Autodesk Inventor part; units mm, degrees
ref_plane "YZ Plane" through (0, 0, 0) normal (1, 0, 0) x (0, 1, 0)
ref_plane "XZ Plane" through (0, 0, 0) normal (0, 1, 0) x (-1, 0, 0)
ref_plane "XY Plane" through (0, 0, 0) normal (0, 0, 1) x (1, 0, 0)
sketch "Sketch1" plane through (0, 0, 0) normal (1, 0, 0) x (0, 1, 0)
  circle A0 centre (0, 0) radius 6
  line L0 (36, -46) -> (36, 34)
  line L1 (36, 34) -> (-29, 34)
  line L2 (-29, 34) -> (-29, -46)
  line L3 (-29, -46) -> (36, -46)
  point P0 (0, -17.5)
  point P1 (17.5, 0)
  point P2 (0, 17.5)
  point P3 (-17.5, 0)
  point P4 (0, -30)
  point P5 (0, 30)
  point P6 (31, -41)
  point P7 (31, 29)
  point P8 (-24, 29)
  point P9 (-24, -41)
  dimension "d6" = 30
  dimension "d9" = 360
  dimension "d15" = 5
  dimension "d16" = 5
  dimension "d17" = 80
  dimension "d18" = 65
  dimension "d28" = 5
  dimension "d29" = 55
  dimension "d30" = 55
  dimension "d38" = 12
extrude "Extrusion1" add sketch "Sketch1" along normal blind 2
hole "Hole1" at (0, 31, -41) at (0, 31, 29) at (0, -24, 29) at (0, -24, -41) direction (1, 0, 0) diameter 3.2 depth 43.75 tip angle 118
sketch "Sketch2" plane through (0, 0, 0) normal (-1, 0, 0) x (0, 0, 1)
  circle A0 centre (-40, 0) radius 6
  line L0 (-46, 36) -> (34, 36)
  line L1 (-46, 36) -> (-52, 36)
  line L2 (-52, 36) -> (-52, -29)
  line L3 (-52, -29) -> (-46, -29)
  line L4 (-46, -29) -> (-46, 36)
  point P0 (0, 0)
  point P1 (0, 25.1294)
  point P2 (0, -32.6005)
  dimension "d31" = 40
  dimension "d32" = 12
  dimension "d33" = 6
extrude "Extrusion2" add sketch "Sketch2" against normal blind 2 contours L4 L3 L2 L1
extrude "Extrusion3" cut sketch "Sketch2" against normal blind 2 contours A0
sketch "Sketch3" plane through (0, 0, 0) normal (-1, 0, 0) x (0, 0, 1)
  line L0 (34, 36) -> (34, -29)
  line L1 (34, 36) -> (46, 36)
  line L2 (46, 36) -> (46, -29)
  line L3 (46, -29) -> (34, -29)
  line L4 (34, -29) -> (34, 36)
  line L5 (-52, 36) -> (-52, -29)
  line L6 (-52, 36) -> (-82, 36)
  line L7 (-82, 36) -> (-82, -29)
  line L8 (-82, -29) -> (-52, -29)
  line L9 (-52, -29) -> (-52, 36)
  circle A0 centre (0, 0) radius 6
  circle A1 centre (0, 0) radius 15.315
  circle A2 centre (-40, 0) radius 6
  circle A3 centre (-40, 0) radius 15.315
  line L10 (-40, 15.315) -> (-90.0791, 8.5618)
  line L11 (-35.9433, -14.768) -> (-79.6302, -20.6591)
  line L12 (0, 15.315) -> (59.9492, 7.4438)
  line L13 (-3.9709, -14.9288) -> (55.9782, -22.7999)
  circle A4 centre (29, 15.315) radius 1.6
  point P0 (-71.9486, -24)
  point P1 (-71.9486, 13.715)
  point P2 (-52, -29)
  dimension "d41" = 30.63
  dimension "d39" = 12
  dimension "d40" = 30
  dimension "d42" = 30.63
  dimension "d43" = 7.68
  dimension "d44" = 0
  dimension "d45" = 7.48
extrude "Extrusion4" add sketch "Sketch3" against normal blind 2 contours L1 L2 L12 L0 | L12 L2 L13 L0 | L13 L2 L3 L0 | L5 L10 L7 L6 | L5 A3 L8 L7 L10 | L5 A3
hole "Hole2" at (0, -24, -71.9486) at (0, 13.715, -71.9486) at (0, 15.315, 29) direction (1, 0, 0) diameter 3.2 depth 43.75 tip angle 118
fillet "Fillet1" radius 8.25 4 edges at (1, 36, -82) (1, -29, -82) (1, -29, 46) (1, 36, 46)
sketch "Sketch4" plane through (0, 0, 0) normal (-1, 0, 0) x (0, 0, 1)
  line L0 (46, -20.75) -> (46, 27.75)
  point P0 (0, 0)
  point P1 (46, 0)
hole "Hole3" at (0, 0, 46) direction (1, 0, 0) diameter 3.2 depth 43.75 tip angle 118
fillet "Fillet2" radius 2 2 edges at (1, 1.6, 46) (1, -1.6, 46)
properties part number "motor" material "アルミニウム 6061"
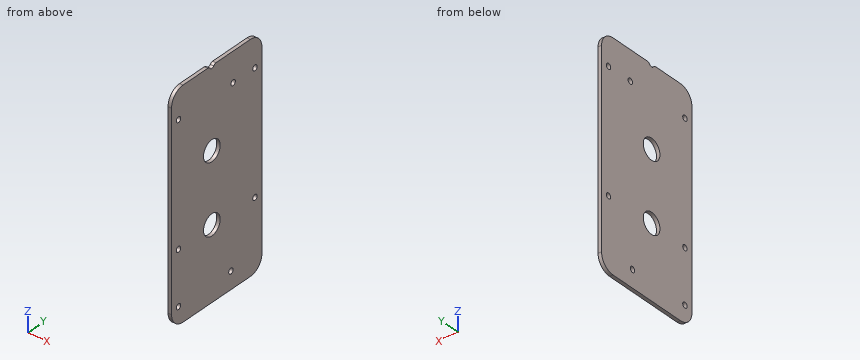
For this review, take the finished solid that the model builds, in its own axes (mm). Give positions to 0.01 mm unless a question says otherwise; leave off trailing zeros. Order: outer loops, then holes, each group sorted by start corner. A loop starts at its lowest first (then second) coordinate and runs counter-clockwise, first axis right, second up. Notation, with made-up numbers: M 6.5,-19 L 21.5,-19 A27 cw 21.5,17 Z; hole C 76.25,-29.5 d6. An arc over 180 degrees is marked long. Answer in a Markdown table with one row per item. Add a question column.
(1) Consider section C-C on y = 31. State the section outline as (x, z) points, and give its area (3 significant figures).
(2) Consider section A-A on z = 29. State the section outline as (x, y) points (3 decimals), and give its area (3 significant figures).
(3) Wall thickness on probe 1 along Y at (x, z) = (1.3, 29) (3 decimals); probe 2 along Z at (x, y) = (1.5, 0); probe 3 along Z at (x, y) = (1, -24): over which ranges is each line inside the solid? List them lowest first. Write a range as [from, to].
(4) Consider section D-D on y = -24. State the section outline as (x, z) points, and give its area (3 significant figures).
(5) Consider section B-B on x = 0.85. Give the number of separate pieces and of enclosed holes in the cut face, and give its area (3 significant figures).
Evaluation:
| question | item | result |
|---|---|---|
| 1 | outline | M 0,-81.33 L 2,-81.33 L 2,-42.6 L 0,-42.6 Z; M 0,-39.4 L 2,-39.4 L 2,27.4 L 0,27.4 Z; M 0,30.6 L 2,30.6 L 2,45.33 L 0,45.33 Z |
| 1 | area | 241 mm^2 |
| 2 | outline | M 0,-29 L 2,-29 L 2,-25.6 L 0,-25.6 Z; M 0,-22.4 L 2,-22.4 L 2,13.715 L 0,13.715 Z; M 0,16.915 L 2,16.915 L 2,29.4 L 0,29.4 Z; M 0,32.6 L 2,32.6 L 2,36 L 0,36 Z |
| 2 | area | 111 mm^2 |
| 3 | probe 1 | y = [-29, -25.6], [-22.4, 13.715], [16.915, 29.4], [32.6, 36] |
| 3 | probe 2 | z = [-82, -46], [-34, -6], [6, 44.4] |
| 3 | probe 3 | z = [-81.33, -73.55], [-70.35, -42.6], [-39.4, 27.4], [30.6, 45.33] |
| 4 | outline | M 0,-81.33 L 2,-81.33 L 2,-73.55 L 0,-73.55 Z; M 0,-70.35 L 2,-70.35 L 2,-42.6 L 0,-42.6 Z; M 0,-39.4 L 2,-39.4 L 2,27.4 L 0,27.4 Z; M 0,30.6 L 2,30.6 L 2,45.33 L 0,45.33 Z |
| 4 | area | 234 mm^2 |
| 5 | separate pieces | 1 |
| 5 | enclosed holes | 9 |
| 5 | area | 7,970 mm^2 |
